Build history of the part. All positions in model axes, mm. A direction names the side the tool comes from. Round coordinates to 2 decimals unless told otherwise and drop trailing zeros. Write each loop counter-clockwise with the first axis right and the second up, starting at its lowest first coordinate (ties: lowest second). Pieces come first, ordered by that corner, then holes. Notation, with made-up numbers: (2.5, 6.25) -> (20.5, 6.25) arc R28 cw to (20.5, 43.25) -> close; hole circle Ø8 at (65, 16). An arc over 180 degrees is marked (long way). Answer in a Markdown table with one row per item.
```python
from build123d import *

# Parameters (mm, degrees)
F0_W      = 140
F0_H      = 41
F1_DEPTH  = 10
F3_R      = 16.5
F4_DEPTH  = 25
F5_R      = 11.5
F6_DEPTH  = 25
F8_R      = 7
F9_R      = 3
F11_DEPTH = 5


with BuildPart() as f1:
    # F0 (on Top) → F1 (new body)
    with BuildSketch(Plane.XY):
        with Locations((-23.8188230246, -17.8435179276)):
            Rectangle(F0_W, F0_H)
    extrude(amount=F1_DEPTH)

    # F3 (on face) → F4 (join)
    with BuildSketch(Plane.XY.offset(10)):
        with Locations((-23.8188230246, -17.8435179276)):
            Circle(F3_R)
    extrude(amount=F4_DEPTH)

    # F5 (on face) → F6 (cut)
    with BuildSketch(Plane.XY.offset(35)):
        with Locations((-23.8188230246, -17.8435179276)):
            Circle(F5_R)
    extrude(amount=-F6_DEPTH, mode=Mode.SUBTRACT)

    # F8
    f8_edges = [f1.edges().sort_by_distance(p)[0] for p in [
        (-93.818823, -38.343518, 5),
        (46.181177, -38.343518, 5),
        (46.181177, 2.656482, 5),
        (-93.818823, 2.656482, 5),
    ]]
    fillet(f8_edges, radius=F8_R)

    # F9
    f9_edges = [f1.edges().sort_by_distance(p)[0] for p in [
        (-23.818823, -38.343518, 10),
    ]]
    fillet(f9_edges, radius=F9_R)

    # F10 (on face) → F11 (join)
    with BuildSketch(Plane.XY.offset(10)):
        with BuildLine():
            ThreePointArc((-23.8188230779, -38.3435179276), (-9.3231340291, -32.3392069607), (-3.3188230246, -17.8435179276))
            ThreePointArc((-3.3188230246, -17.8435179276), (-9.3231340103, -3.3478289133), (-23.8188230246, 2.6564820724))
            ThreePointArc((-23.8188230246, 2.6564820724), (-44.3188230246, -17.843517901), (-23.8188230779, -38.3435179276))
        make_face()
    extrude(amount=-F11_DEPTH)


solid = f1.part
```
Q1. Wall check: line 1 (Z direction, x = 8.5, y = -30.5); line 2 (X direction, y = -26.5, z = 23.5); line 3 (X direction, y = -25, z = 30). Give the ranges that are in metal, low to high. Write a range as [from, to].
A:
| item | result |
|---|---|
| line 1 | [0, 10] |
| line 2 | [-37.87, -31.39], [-16.25, -9.77] |
| line 3 | [-38.69, -32.82], [-14.82, -8.95] |
Q2. Saw through at A-A on x = 20. Write the cut outline in (y, z).
A:
| item | result |
|---|---|
| outline | (-38.34, 0) -> (2.66, 0) -> (2.66, 7) arc R3 ccw to (-0.34, 10) -> (-35.34, 10) arc R3 ccw to (-38.34, 7) -> close |
Q3. Saw through at B-B on y = -10. Write the cut outline in (x, z), plus the area to 3 significant figures.
A:
| item | result |
|---|---|
| outline | (-93.82, 0) -> (46.18, 0) -> (46.18, 7) arc R3 ccw to (43.18, 10) -> (-9.3, 10) -> (-9.3, 35) -> (-15.41, 35) -> (-15.41, 10) -> (-32.23, 10) -> (-32.23, 35) -> (-38.34, 35) -> (-38.34, 10) -> (-90.82, 10) arc R3 ccw to (-93.82, 7) -> close |
| area | 1,700 mm² |
Q4. Saw through at D-D on x = -16.5. Write the cut outline in (y, z), plus the area to 3 significant figures.
A:
| item | result |
|---|---|
| outline | (-38.34, 0) -> (2.66, 0) -> (2.66, 7) arc R3 ccw to (1.31, 9.51) -> (1.31, 10) -> (-3.06, 10) -> (-3.06, 35) -> (-8.97, 35) -> (-8.97, 10) -> (-26.71, 10) -> (-26.71, 35) -> (-32.63, 35) -> (-32.63, 10) -> (-36.99, 10) -> (-36.99, 9.51) arc R3 ccw to (-38.34, 7) -> close |
| area | 703 mm² |
Q5. Two-plate mould, pull along X, no slides. Class faces 4 (the cylindrical face through (-36.9, -27.9, 22.3)), 5 (the cylindrical face through (-25.32, -6.44, 22.68)), 6 (the cylindrical face through (45.279, -17.655, 9.145)): released by +X, released by -X, zero draft, split by the parting line, or undercut.
A:
| item | result |
|---|---|
| face 4 | split by the parting line |
| face 5 | undercut |
| face 6 | released by +X |
Q6. Drop flat-ended pins along their axis: P1, Ø12, axis at y = -3.5, z = 16.5, coming from the -X side; P2, Ø14, axis at x = -23.82, y = -17.84, coming from the +Z side; P3, Ø12, axis at y = -18, z = 14, coming from the -X side; P4, Ø12, axis at x = -17.5, y = -24.5, coming from the +Z side. Give the stop position or say it passes through.
A:
| item | result |
|---|---|
| P1 | x = -38.05 |
| P2 | z = 10 |
| P3 | x = -93.65 |
| P4 | z = 35 |
Q7. Saw through at C-C on z = 16. Write the cut outline in (x, y), plus the area to 3 significant figures.
A:
| item | result |
|---|---|
| outline | circle Ø33 at (-23.82, -17.84); hole circle Ø23 at (-23.82, -17.84) |
| area | 440 mm² |
Q8. Which spindle directions (+Z, -Z, +X, -X, +Y, -Y) get a long thin tool onto all of the face, cutting with end or side? Do faces 1 (the cylindrical face through (8.122, -37.441, 9.145)), 2 (the cylindrical face through (-55.8, 1.8, 9.1)), 3 (the cylindrical face through (7.2, 1.8, 9.1)). Say none if no direction does.
A:
| item | result |
|---|---|
| face 1 | +Z, +X, -Y |
| face 2 | +Z, -X, +Y |
| face 3 | +Z, +X, +Y |
